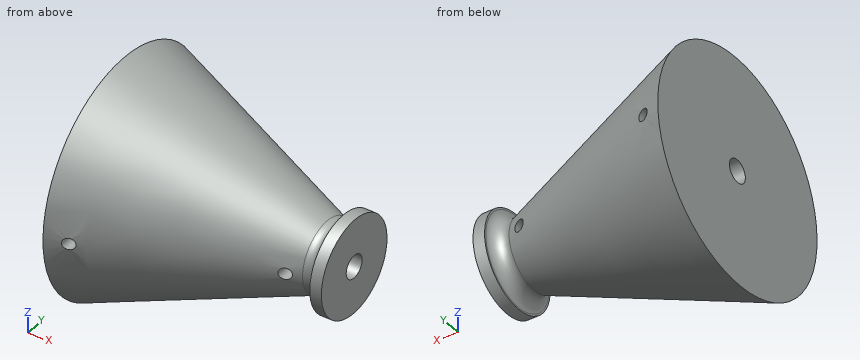
```python
from build123d import *

# Parameters (mm, degrees)
F2_R          = 1
F3_R          = 0.5
F4_DEPTH      = 10.001
F4_DEPTH_BACK = 10.001


with BuildPart() as f1:
    # F0 (on Front) → F1 (revolve)
    with BuildSketch(Plane.XZ):
        Polygon((0, 10), (0, 1), (20, 1), (20, 4.1248017436), (19, 4.1248017436), (19, 2.5), align=None)
    revolve(axis=Axis((8.1747960717, 0, 0), (1, 0, 0)))

    # F2
    f2_edges = [f1.edges().sort_by_distance(p)[0] for p in [
        (19, 0, -2.5),
    ]]
    fillet(f2_edges, radius=F2_R)

    # F3 (on Front) → F4 (cut, two sides)
    with BuildSketch(Plane.XZ) as f4_sk:
        with Locations((1.7530444311, 0)):
            Circle(F3_R)
        with Locations((16.452120617, 0)):
            Circle(F3_R)
    extrude(amount=-F4_DEPTH, mode=Mode.SUBTRACT)
    extrude(f4_sk.sketch, amount=F4_DEPTH_BACK, mode=Mode.SUBTRACT)


solid = f1.part
```
CAD build for the part. Positions are in the model's coordinates, mm. Round coordinates to 2 decimals unless told otherwise and drop trailing zeros. Order: outer loops, then holes, each group sorted by start corner. A loop starts at its lowest first (then second) coordinate and runs counter-clockwise, first axis right, second up. Notation, with made-up numbers: (7.5, 67) - (35.5, 67) arc R15 cw to (35.5, 79) - close; hole circle Ø5 at (11, -34). An arc over 180 degrees is marked (long way). Use CSV: the item, a comma, the result in double quotes. Start each with the question number.
1) Saw through at A-A (z = 0). Count the separate pieces of the cut face and the enclosed holes in it, and give its area (3 significant figures).
2) Saw through at C-C (x = 5.5). List the corners of the cut face in (y, z).
3) Pin check, flat tips, straight feed: pin 1 Ø6 at (x, y) = (4.5, -4.5) entering from +Z; pin 2 Ø5 at (x, z) = (3.5, -2) entering from -Y; pin 3 Ø3 at (x, y) = (12.5, 2) entering from -Z; pin 4 Ø1.6 at (y, z) = (0, 0) entering from -X. Stop position of each tip, or through.
4) Saw through at B-B (y = 0). List the corners of the cut face in (x, z), and give its area (3 significant figures).
5) Wall check: L1, parallel to X at y = -2, z = 0; L2, parallel to Z at x = 19.25, y = 0; L3, parallel to Z at x = 14.75, y = 0. Give the ranges that are in metal, low to high. Write a range as [from, to].
Values follow:
1,separate pieces,"6"
1,enclosed holes,"0"
1,area,"185 mm2"
2,outline,"circle Ø15.66 at (0, 0); hole circle Ø2 at (0, 0)"
3,pin 1,"stops at z = 8.76"
3,pin 2,"stops at y = -9.48"
3,pin 3,"stops at z = -5.44"
3,pin 4,"passes through"
4,outline,"(0, -10) - (17.63, -3.04) arc R1 cw to (19, -3.97) - (19, -4.12) - (20, -4.12) - (20, -1) - (0, -1) - close; (0, 1) - (20, 1) - (20, 4.12) - (19, 4.12) - (19, 3.97) arc R1 cw to (17.63, 3.04) - (0, 10) - close"
4,area,"207 mm2"
5,L1,"x = [0, 1.25], [2.25, 15.95], [16.95, 20]"
5,L2,"z = [-4.12, -1], [1, 4.12]"
5,L3,"z = [-4.18, -1], [1, 4.18]"
